Here's the drawing with two shaded views (mm, measured from the low corner). I have some questions. A direction names the side the tool comes from. Coordinates: 2 decimals unless noted, no trailing zeros. Loops run counter-clockwise (first coordinate to the right, second up) from the corner with the lowest first, then second, coordinate; pieces in that order, holes last. Notation, with made-up numbers: (9.5, -37.75) -> (49.5, -37.75) arc R19 ccw to (49.5, -29.75) -> close; hole circle Ø4 at (-34, 52.25). An arc over 180 degrees is marked (long way). Use CSV: the item, a comma, the result in double quotes. Start each with the question number.
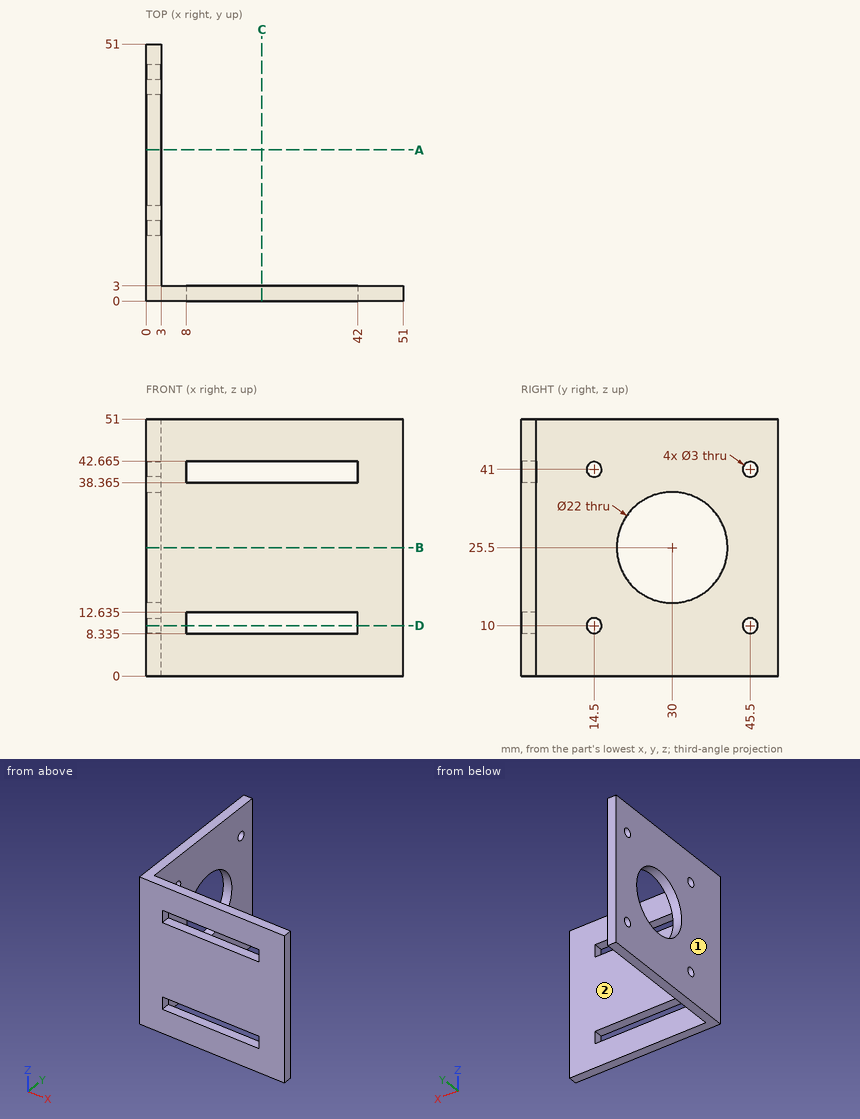
1) I want a section at D-D, the plane z = 10. Please give me the cut outline in (x, y).
2) I want a section at C-C, the plane x = 23. Please give me the cut outline in (y, z) (3 decimals), plus the area to 3 significant figures.
3) For P1, Ø17.5, axis at y = 30, z = 25.5, coming from the +X side; P2, Ø24, axis at y = 28.5, z = 19, coming from the +X side; P3, Ø2, axis at x = 45.5, z = 11.5, coming from the +Y side, each with a flat end and sliding along its axis, tell me the tip position at first contact or that it passes through.
4) Which directions (+Z, -Z, +X, -X, +Y, -Y) give clear straight access to the entire face, cutting with the end or side of a thin tool? Please do the marked faces 1 and 2.
5) Please list where these lines run through material, in increasing order: L1, parallel to Y at x = 1.4, z = 10; L2, parallel to Y at x = 0.9, z = 25.5; L3, parallel to Y at x = 20, z = 44. Write a range as [from, to].
6) I want a section at A-A, the plane y = 30. Please give me the cut outline in (x, z), plus the area to 3 significant figures.
7) I want a section at B-B, the plane z = 25.5. Please give me the cut outline in (x, y), plus the area to 3 significant figures.
Return value:
1,outline,"(0, 0) -> (8, 0) -> (8, 3) -> (3, 3) -> (3, 13) -> (0, 13) -> close; (0, 16) -> (3, 16) -> (3, 44) -> (0, 44) -> close; (0, 47) -> (3, 47) -> (3, 51) -> (0, 51) -> close; (42, 0) -> (51, 0) -> (51, 3) -> (42, 3) -> close"
2,outline,"(0, 0) -> (3, 0) -> (3, 8.335) -> (0, 8.335) -> close; (0, 12.635) -> (3, 12.635) -> (3, 38.365) -> (0, 38.365) -> close; (0, 42.665) -> (3, 42.665) -> (3, 51) -> (0, 51) -> close"
2,area,"127 mm²"
3,P1,"passes through"
3,P2,"stops at x = 3"
3,P3,"stops at y = 3"
4,face 1,"+Z, -Z, -X, +Y, -Y"
4,face 2,"+Z, -Z, +X, +Y"
5,L1,"y = [0, 13], [16, 44], [47, 51]"
5,L2,"y = [0, 19], [41, 51]"
5,L3,"y = [0, 3]"
6,outline,"(0, 0) -> (3, 0) -> (3, 14.5) -> (0, 14.5) -> close; (0, 36.5) -> (3, 36.5) -> (3, 51) -> (0, 51) -> close"
6,area,"87.0 mm²"
7,outline,"(0, 0) -> (51, 0) -> (51, 3) -> (3, 3) -> (3, 19) -> (0, 19) -> close; (0, 41) -> (3, 41) -> (3, 51) -> (0, 51) -> close"
7,area,"231 mm²"
